Source: CAD feature listing. Evaluate the final solid. Frame: model axes, mm. A direction names the side the tool comes from. Coordinates: 2 decimals unless noted, no trailing zeros. Order: outer loops, then holes, each group sorted by start corner. A loop starts at its lowest first (then second) coordinate and runs counter-clockwise, first axis right, second up. Notation, with made-up numbers: (-8, 51) -> (49, 51) arc R3 ccw to (49, 56) -> close; hole circle Ø11 at (0, -31). An arc over 180 degrees is marked (long way). Put each result on its own line as item: value.
from build123d import *

# Parameters (mm, degrees)
SKETCH1_W               = 54.991
SKETCH1_H               = 26.289
SKETCH1_R               = 1.5875
SKETCH1_W_2             = 39.751
SKETCH1_H_2             = 18.669
BASE_DEPTH              = 2.54
SKETCH2_W               = 54.991
SKETCH2_H               = 3.81
F_4_HOLE_DEPTH          = 20.32
SKETCH3_W               = 42.291
SKETCH3_H               = 20.32
GAP_DEPTH               = 64.65449805
FILLET1_R               = 2.54
CHAMFER1_SIZE           = 1.27
SKETCH4_R               = 1.4605
SERVO_SCREW_HOLES_DEPTH = 64.65449805


with BuildPart() as part:
    # Sketch1 → Base (new body)
    with BuildSketch(Plane(origin=(0, 0, 0), x_dir=(1, 0, 0), z_dir=(0, 1, 0))):
        with Locations((27.4955, 13.1445)):
            Rectangle(SKETCH1_W, SKETCH1_H)
        with Locations(Location((51.6255, 13.1445, 0), (0, 0, 270))):
            Circle(SKETCH1_R, mode=Mode.SUBTRACT)
        with Locations(Location((3.3655, 13.1445, 0), (0, 0, 270))):
            Circle(SKETCH1_R, mode=Mode.SUBTRACT)
        with Locations((27.4955, 13.1445)):
            Rectangle(SKETCH1_W_2, SKETCH1_H_2, mode=Mode.SUBTRACT)
    extrude(amount=BASE_DEPTH)

    # Sketch2 → 4 hole (add)
    with BuildSketch(Plane(origin=(0, 2.54, 0), x_dir=(1, 0, 0), z_dir=(0, 1, 0))):
        with Locations((27.4955, 24.384)):
            Rectangle(SKETCH2_W, SKETCH2_H)
    extrude(amount=F_4_HOLE_DEPTH)

    # Sketch3 → gap (cut, through all)
    with BuildSketch(Plane.XY.offset(-22.479)):
        with Locations((27.4955, 12.7)):
            Rectangle(SKETCH3_W, SKETCH3_H)
    extrude(amount=-GAP_DEPTH, mode=Mode.SUBTRACT)

    # Fillet1
    fillet1_edges = [part.edges().sort_by_distance(p)[0] for p in [
        (0, 22.86, -24.384),
        (54.991, 22.86, -24.384),
        (6.35, 22.86, -24.384),
        (48.641, 22.86, -24.384),
        (54.991, 1.27, 0),
        (0, 1.27, 0),
    ]]
    fillet(fillet1_edges, radius=FILLET1_R)

    # Chamfer1
    chamfer1_edges = [part.edges().sort_by_distance(p)[0] for p in [
        (51.6255, 2.54, -14.732),
        (3.3655, 2.54, -14.732),
    ]]
    chamfer(chamfer1_edges, length=CHAMFER1_SIZE)

    # Sketch4 → servo screw holes (cut, through all)
    with BuildSketch(Plane.XY.offset(-22.479)):
        with Locations((3.175, 17.5895)):
            Circle(SKETCH4_R)
        with Locations((3.175, 7.0485)):
            Circle(SKETCH4_R)
        with Locations((51.816, 17.5895)):
            Circle(SKETCH4_R)
        with Locations((51.816, 7.0485)):
            Circle(SKETCH4_R)
    extrude(amount=-SERVO_SCREW_HOLES_DEPTH, mode=Mode.SUBTRACT)


solid = part.part
1. Ray query, line 1 along Z through (x, y) = (23.5, 1.5); line 2 along X through (y, z) = (2.25, -10.25); line 3 along Y through (x, z) = (4.5, -21.75). Return the intervals inside material, ascending.
Numbers:
line 1: z = -26.29 to -22.48, -3.81 to 0
line 2: x = 0 to 7.62, 47.37 to 54.99
line 3: y = 0 to 2.54
2. Pull-direction query (Y, two-part tool) for faces 6 (the flat face through (3, 13, -22.479)), 7 (the cylindrical face through (52.6, 18.82, -24.36)), 8 (the flat face through (52, 22.86, -24)); classes: pulls with the +Y half, pulls with the -Y half, needs draft (parallel to the pull), parting line crosses it, or undercut.
Numbers:
face 6: needs draft
face 7: undercut
face 8: pulls with the +Y half
3. Set-up query: faces 1 (the flat face through (27, 1, -22.479)), 2 (the flat face through (52, 13, -22.479)), 3 (the flat face through (6.35, 11, -24)), 4 (the flat face through (3, 22.86, -24)), 5 (the flat face through (27, 0, -2)). Return all of +Z, -Z, +X, -X, +Y, -Y with unobstructed straight access to the full face (end or side cutting, diameter ignored); none if empty.
Numbers:
face 1: +Y, -Y
face 2: +Z, +X, -X, +Y
face 3: +Z, -Z, +Y
face 4: +Z, -Z, +X, -X, +Y
face 5: +Z, -Z, +X, -X, -Y
4. Cut plane D-D on y = 2. Output: boundary loops of the cut face in (x, z) (1 decimal).
Numbers:
outline: (0, -26.3) -> (55, -26.3) -> (55, -2.5) arc R2.5 ccw to (52.5, 0) -> (2.5, 0) arc R2.5 ccw to (0, -2.5) -> close; hole circle Ø4.6 at (3.4, -13.1); hole (7.6, -22.5) -> (47.4, -22.5) -> (47.4, -3.8) -> (7.6, -3.8) -> close; hole circle Ø4.6 at (51.6, -13.1)
5. First-contact query: pin 1 (2 mm diameter, centred on x = 45.5, z = -10, fed in from +Y); pin 2 (5 mm diameter, centred on x = 3.5, y = 15, fed in from +Z). Flat tips, straight axial feed; report the tip coordinate or a pass-through.
Numbers:
pin 1: passes through
pin 2: stops at z = -22.48
6. Cut plane C-C on y = 17. Output: boundary loops of the cut face in (x, z), plus the area to 3 significant figures.
Numbers:
outline: (0, -26.29) -> (1.84, -26.29) -> (1.84, -22.48) -> (0, -22.48) -> close; (4.51, -26.29) -> (6.35, -26.29) -> (6.35, -22.48) -> (4.51, -22.48) -> close; (48.64, -26.29) -> (50.48, -26.29) -> (50.48, -22.48) -> (48.64, -22.48) -> close; (53.15, -26.29) -> (54.99, -26.29) -> (54.99, -22.48) -> (53.15, -22.48) -> close
area: 28.0 mm2
7. Cut plane B-B on z = -6.5. Output: boundary loops of the cut face in (x, y).
Numbers:
outline: (0, 0) -> (7.62, 0) -> (7.62, 2.54) -> (0, 2.54) -> close; (47.37, 0) -> (54.99, 0) -> (54.99, 2.54) -> (47.37, 2.54) -> close
8. Cut plane A-A on x = 34. Output: boundary loops of the cut face in (y, z), plus the area to 3 significant figures.
Numbers:
outline: (0, -26.29) -> (2.54, -26.29) -> (2.54, -22.48) -> (0, -22.48) -> close; (0, -3.81) -> (2.54, -3.81) -> (2.54, 0) -> (0, 0) -> close
area: 19.4 mm2
